Read the model definition and answer for the solid it produces. Units are mm, in the model's axes. Face numbers are marked on the shaded views. A direction names the side the tool comes from. Coordinates: 2 decimals unless noted, no trailing zeros. Order: outer loops, then holes, each group sorted by start corner. A loop starts at its lowest first (then second) coordinate and runs counter-clockwise, first axis right, second up. Notation, with made-up numbers: M 84,45.25 L 92,45.25 A22 cw 92,61.25 Z; hole C 62.5,70 d4. An arc over 180 degrees is marked long. One line per question, with ' | ' between items. Start each with the question number.
1) A tool of negligible diameter and unlimited length cuts with its end or side. For the marked faces 4 and 5, from which of +Z, -Z, +X, -X, +Y, -Y can it reach the whole face along a straight path? Write none if from no direction.
2) Consider probe 1 along Y at (x, z) = (-13, 14); probe 2 along Z at (x, y) = (0, -37.5); probe 3 along X at (y, z) = (-32.5, 6.5). Determine where each line is inside the solid, lowest interval first.
3) Find section C-C, the plane y = 2.5. Write down the section's boundary in (x, z), plus the area to 3 significant figures.
4) Find section D-D, the plane z = 7. Write down the section's boundary in (x, y).
5) Given P1, Ø1, axis at x = -10.5, y = -19, coming from the +Z side; P2, Ø6.5, axis at x = -10, z = 7, coming from the -Y side; P3, Ø0.5, axis at y = 36, z = 15.5, coming from the -X side; P4, Ø0.7, axis at y = -36.5, z = 15.5, coming from the +X side, each flat-ended and moving along its own axis, determine where each tip first touches the part or whether it passes through.
6) Find section B-B, the plane z = 13.75. Write down the section's boundary in (x, y), plus the area to 3 significant figures.
7) Find section A-A, the plane x = 0. Write down the section's boundary in (y, z).
8) The mould has two halves that part along X. Classify the marked faces 1, 2 and 3: +X half, -X half, draft (parallel to the pull), parting line (faces both ways), or undercut.
from build123d import *

# Parameters (mm, degrees)
F0_W     = 40
F0_H     = 78
F1_DEPTH = 16
F2_R     = 2
F3_T     = -2.2
F4_R     = 2.5
F5_DEPTH = 2.2
F7_DEPTH = 12.5
F8_SIZE  = 1


with BuildPart() as f1:
    # F0 (on Top) → F1 (new body)
    with BuildSketch(Plane.XY):
        Rectangle(F0_W, F0_H)
    extrude(amount=F1_DEPTH)

    # F2
    f2_edges = [f1.edges().sort_by_distance(p)[0] for p in [
        (-20, -39, 8),
        (20, -39, 8),
        (-20, 39, 8),
        (20, 39, 8),
    ]]
    fillet(f2_edges, radius=F2_R)

    # F3
    f3_openings = [f1.faces().sort_by_distance(p)[0] for p in [
        (0, 0, 16),
    ]]
    offset(amount=F3_T, openings=f3_openings)

    # F4 (on face) → F5 (cut, through all)
    with BuildSketch(Plane.XZ.offset(39)):
        with Locations((-10, 7)):
            Circle(F4_R)
        with Locations((0, 7)):
            Circle(F4_R)
        with Locations((10, 7)):
            Circle(F4_R)
    extrude(amount=-F5_DEPTH, mode=Mode.SUBTRACT)

    # F6 (on Right) → F7 (join, symmetric)
    with BuildSketch(Plane.YZ):
        Polygon((-36.8, 16), (-36.8, 15.1609003688), (-35.8, 16), align=None)
        Polygon((35.3, 16), (36.8, 14.9496886927), (36.8, 16), align=None)
    extrude(amount=F7_DEPTH, both=True)

    # F8
    f8_edges = [f1.edges().sort_by_distance(p)[0] for p in [
        (0, -39, 16),
    ]]
    chamfer(f8_edges, length=F8_SIZE)


solid = f1.part
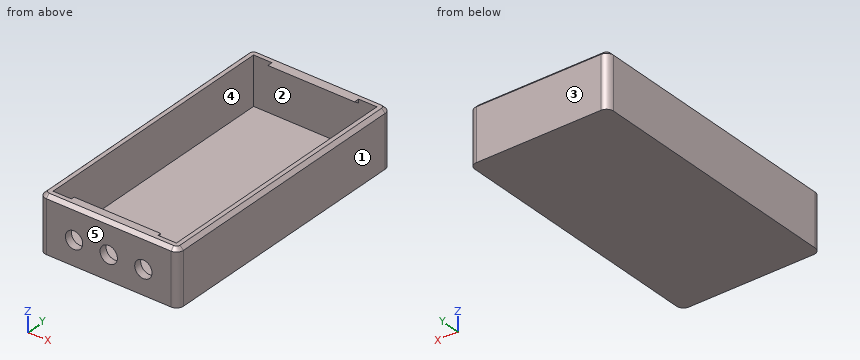
Report:
1) face 4: +Z | face 5: +Z, -Z, +X, -X, -Y
2) probe 1: y = -39 to -36.8, 36.8 to 39 | probe 2: z = 0 to 4.5, 9.5 to 16 | probe 3: x = -20 to -17.8, 17.8 to 20
3) outline: M -20,0 L 20,0 L 20,15 L 19,16 L 17.8,16 L 17.8,2.2 L -17.8,2.2 L -17.8,16 L -19,16 L -20,15 Z | area: 148 mm^2
4) outline: M -20,-37 A2 ccw -18,-39 L -12.5,-39 L -12.5,-36.8 L -17.8,-36.8 L -17.8,36.8 L 17.8,36.8 L 17.8,-36.8 L 12.5,-36.8 L 12.5,-39 L 18,-39 A2 ccw 20,-37 L 20,37 A2 ccw 18,39 L -18,39 A2 ccw -20,37 Z; M -7.5,-39 L -2.5,-39 L -2.5,-36.8 L -7.5,-36.8 Z; M 2.5,-39 L 7.5,-39 L 7.5,-36.8 L 2.5,-36.8 Z
5) P1: stops at z = 2.2 | P2: stops at y = -39 | P3: stops at x = -19.75 | P4: stops at x = 19.85
6) outline: M -20,-37 A2 ccw -18,-39 L 18,-39 A2 ccw 20,-37 L 20,37 A2 ccw 18,39 L -18,39 A2 ccw -20,37 Z; hole M -17.8,-36.8 L 17.8,-36.8 L 17.8,36.8 L -17.8,36.8 Z | area: 496 mm^2
7) outline: M -39,0 L 39,0 L 39,15 L 38,16 L 35.3,16 L 36.8,14.95 L 36.8,2.2 L -36.8,2.2 L -36.8,4.5 L -39,4.5 Z; M -39,9.5 L -36.8,9.5 L -36.8,15.16 L -35.8,16 L -38,16 L -39,15 Z
8) face 1: +X half | face 2: undercut | face 3: draft
